Geometry: final body of the model. Coordinates: model frame, mm. Face numbers are marked on the shaded views. A direction names the side the tool comes from. Round coordinates to 2 decimals unless told otherwise and drop trailing zeros. Loops run counter-clockwise (first coordinate to the right, second up) from the corner with the lowest first, then second, coordinate; pieces in that order, holes last. Notation, with made-up numbers: (-19.75, 54) - (39.25, 54) arc R7 ccw to (39.25, 64) - close; hole circle Ø7 at (0.5, 0). An arc over 180 degrees is marked (long way). Answer in a Markdown table with one row per item. Add a question column.
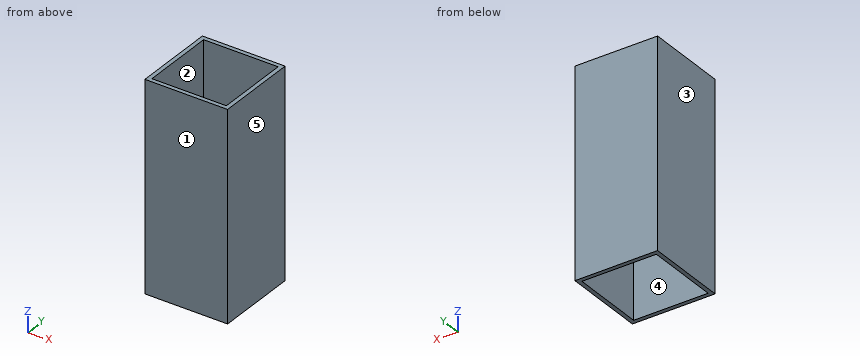
from build123d import *

# Parameters (mm, degrees)
F0_W     = 50.8
F0_H     = 50.8
F1_DEPTH = 63.5
F2_T     = -2.54


with BuildPart() as f1:
    # F0 (on Top) → F1 (new body, symmetric)
    with BuildSketch(Plane.XY):
        Rectangle(F0_W, F0_H)
    extrude(amount=F1_DEPTH, both=True)

    # F2
    f2_openings = [f1.faces().sort_by_distance(p)[0] for p in [
        (0, 0, 63.5),
        (0, 0, -63.5),
    ]]
    offset(amount=F2_T, openings=f2_openings)


solid = f1.part
1) Reachability of the marked faces 4 and 5 from +Z, -Z, +X, -X, +Y, -Y: full face, straight path, thin tool, end or side. Return the list, or none.
2) Material intervals for line 1 along Y through (x, z) = (5.5, 18.5), sorted ascending. Write a range as from..to.
3) Section A-A, the plane y = -2.5. Return the cut outline in (x, z).
4) Pull-direction query (X, two-part tool) for the marked faces 1, 2 and 3; classes: pulls with the +X half, pulls with the -X half, needs draft (parallel to the pull), parting line crosses it, or undercut.
5) Section C-C, the plane z = -49. Return the cut outline in (x, y).
Evaluation:
| question | item | result |
|---|---|---|
| 1 | face 4 | +Z, -Z |
| 1 | face 5 | +Z, -Z, +X, +Y, -Y |
| 2 | line 1 | y = -25.4..-22.86, 22.86..25.4 |
| 3 | outline | (-25.4, -63.5) - (-22.86, -63.5) - (-22.86, 63.5) - (-25.4, 63.5) - close; (22.86, -63.5) - (25.4, -63.5) - (25.4, 63.5) - (22.86, 63.5) - close |
| 4 | face 1 | needs draft |
| 4 | face 2 | undercut |
| 4 | face 3 | pulls with the -X half |
| 5 | outline | (-25.4, -25.4) - (25.4, -25.4) - (25.4, 25.4) - (-25.4, 25.4) - close; hole (-22.86, -22.86) - (22.86, -22.86) - (22.86, 22.86) - (-22.86, 22.86) - close |
